from build123d import *

# Parameters (mm, degrees)
F0_W     = 119.38
F0_H     = 84.3915
F1_DEPTH = 6.35
F2_W     = 119.38
F2_H     = 84.3915
F3_DEPTH = 9.525
F4_R     = 1.5875
F5_DEPTH = 4.7625


with BuildPart() as f1:
    # F0 (on Top) → F1 (new body)
    with BuildSketch(Plane.XY):
        Polygon((-47.6464699149, 94.2441691224), (-53.9964699149, 94.2441691224), (-53.9964699149, -2.8473308776), (78.0835300851, -2.8473308776), (78.0835300851, 0), (78.0835300851, 94.2441691224), align=None)
        with Locations((12.0435300851, 45.6984191224)):
            Rectangle(F0_W, F0_H, mode=Mode.SUBTRACT)
        with Locations((12.0435300851, 45.6984191224)):
            Rectangle(F0_W, F0_H)
    extrude(amount=F1_DEPTH)

    # F2 (on face) → F3 (join)
    with BuildSketch(Plane.XY.offset(6.35)):
        Polygon((71.7335300851, 94.2441691224), (-53.9964699149, 94.2441691224), (-53.9964699149, 87.8941691224), (-53.9964699149, -2.8473308776), (-47.6464699149, -2.8473308776), (78.0835300851, -2.8473308776), (78.0835300851, 3.5026691224), (78.0835300851, 94.2441691224), align=None)
        with Locations((12.0435300851, 45.6984191224)):
            Rectangle(F2_W, F2_H, mode=Mode.SUBTRACT)
    extrude(amount=F3_DEPTH)

    # F4 (on face) → F5 (join)
    with BuildSketch(Plane.XY.offset(6.35)):
        with Locations((32.3635300851, 81.3854191224)):
            Circle(F4_R)
        with Locations((60.3035300851, 81.3854191224)):
            Circle(F4_R)
        with Locations((17.1235300851, 22.7114191224)):
            Circle(F4_R)
        with BuildLine():
            ThreePointArc((65.3835300851, 19.8539191224), (66.5060621002, 20.3188871073), (66.9710300851, 21.4414191224))
            ThreePointArc((66.9710300851, 21.4414191224), (64.26099807, 22.5639511376), (65.3835300851, 19.8539191224))
        make_face()
    extrude(amount=F5_DEPTH)


solid = f1.part
Build history of the part. All positions in model axes, mm. A direction names the side the tool comes from. Coordinates: 2 decimals unless noted, no trailing zeros. Order: outer loops, then holes, each group sorted by start corner. A loop starts at its lowest first (then second) coordinate and runs counter-clockwise, first axis right, second up. Notation, with made-up numbers: (-9, 88) - (11, 88) arc R23 ccw to (11, 100) - close; hole circle Ø4 at (-31, 9.5). An arc over 180 degrees is marked (long way). Write item = value, one per line. Start each with the question number.
1) Flat gauge pins, fed straight in: pin 1 Ø1.6 at (x, y) = (65, 21.5) entering from +Z; pin 2 Ø3 at (x, y) = (-40.5, 55.5) entering from +Z. Where does each tip first touch, or does it go through?
2) Wall check: line 1 along Y through (x, z) = (-19.5, 9); line 2 along X through (y, z) = (75, 12.5); line 3 along Z through (x, y) = (66.5, 61). Give the ranges that are in metal, low to high. Write a range as from..to.
3) 3-axis set-ups, long thin cutter, end or side, ignore diameter. For faces 1 (the face through (71.734, 45, 11)), 2 (the face through (11, 46, 0)): which of +Z, -Z, +X, -X, +Y, -Y reach the whole face in a straight line?
4) Saw through at A-A on z = 9.25. Write the cut outline in (x, y) (1 decimal), then the cut area to 3 significant figures.
5) Saw through at C-C on y = 67. Write the cut outline in (x, z) (3 decimals), then the cut area to 3 significant figures.
6) Two-plate mould, pull along X, no slides. Class faces 3 (the face through (17, 23, 11.112)), 4 (the face through (78.084, 45, 8)), 5 (the face through (11, -2.847, 8)), 6 (the face through (60.1, 82.96, 8.7)): pulls with the +X half, pulls with the -X half, needs draft (parallel to the pull), parting line crosses it, or undercut.
7) Saw through at B-B on x = 39.5. Write the cut outline in (y, z) (3 decimals).
From the geometry:
q1.pin_1 = 11.11
q1.pin_2 = 6.35
q2.line_1 = -2.85..3.5, 87.89..94.24
q2.line_2 = -54..-47.65, 71.73..78.08
q2.line_3 = 0..6.35
q3.face_1 = +Z
q3.face_2 = -Z, +X, -X, +Y, -Y
q4.outline = (-54, -2.8) - (78.1, -2.8) - (78.1, 94.2) - (-54, 94.2) - close; circle Ø3.2 at (17.1, 22.7); circle Ø3.2 at (32.4, 81.4); circle Ø3.2 at (60.3, 81.4); circle Ø3.2 at (65.4, 21.4); hole (-47.6, 3.5) - (71.7, 3.5) - (71.7, 87.9) - (-47.6, 87.9) - close
q4.area = 2,780 mm^2
q5.outline = (-53.996, 0) - (78.084, 0) - (78.084, 15.875) - (71.734, 15.875) - (71.734, 6.35) - (-47.646, 6.35) - (-47.646, 15.875) - (-53.996, 15.875) - close
q5.area = 960 mm^2
q6.face_3 = undercut
q6.face_4 = pulls with the +X half
q6.face_5 = needs draft
q6.face_6 = undercut
q7.outline = (-2.847, 0) - (94.244, 0) - (94.244, 15.875) - (87.894, 15.875) - (87.894, 6.35) - (3.503, 6.35) - (3.503, 15.875) - (-2.847, 15.875) - close
